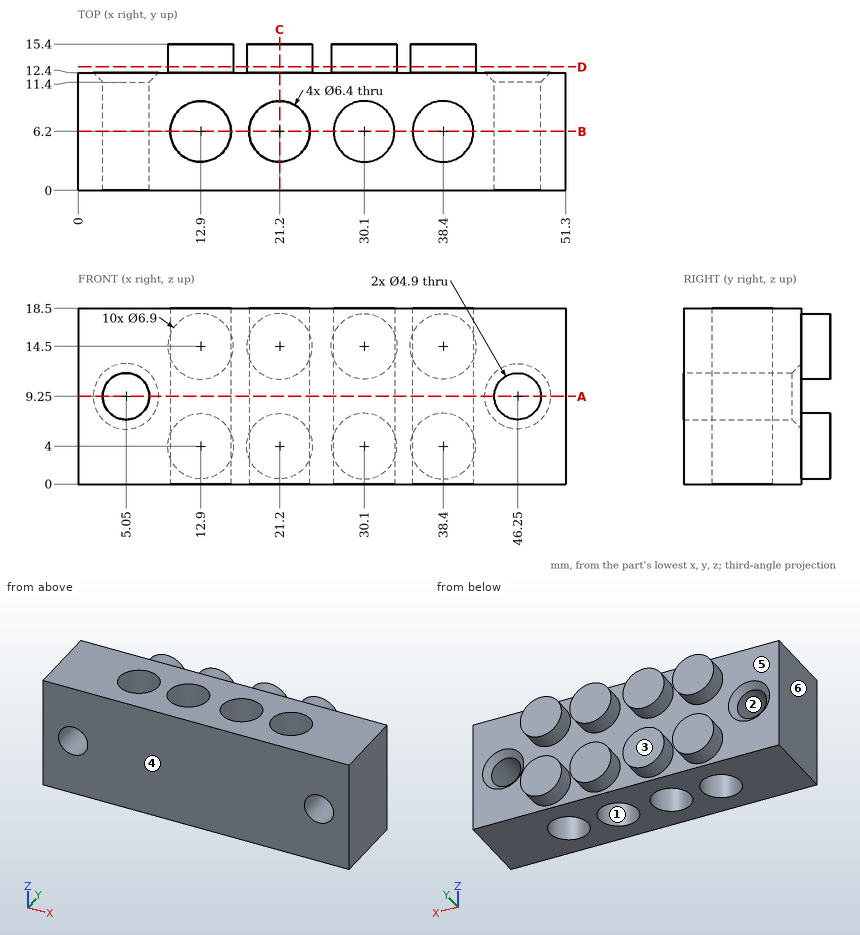
Study the drawing (mm; zero at the part's minimum x, y, z) and answer. A direction names the side the tool comes from. Coordinates: 2 decimals unless noted, no trailing zeros. Write each loop counter-clockwise with the first axis right and the second up, starting at its lowest first coordinate (ties: lowest second). Pieces come first, ordered by that corner, then holes. Notation, with made-up numbers: (21.25, -18.5) -> (71.25, -18.5) arc R12 cw to (71.25, -4.5) -> close; hole circle Ø8 at (35.25, 28). An arc over 180 degrees is marked (long way). Write item = value, one per line.
(1) Section D-D on y = 13 is taken. Write down the section's boundary in (x, z).
From the geometry:
outline = circle Ø6.9 at (12.9, 4); circle Ø6.9 at (12.9, 14.5); circle Ø6.9 at (21.2, 4); circle Ø6.9 at (21.2, 14.5); circle Ø6.9 at (30.1, 4); circle Ø6.9 at (30.1, 14.5); circle Ø6.9 at (38.4, 4); circle Ø6.9 at (38.4, 14.5)
(2) For a pull along Y with two mould halves and no side action, classify the marked faces 1, 2, 3 and 4 as +Y half, -Y half, draft (parallel to the pull), parting line (faces both ways), or undercut.
From the geometry:
face_1 = undercut
face_2 = draft
face_3 = +Y half
face_4 = -Y half
(3) Section C-C on x = 21.2 is taken. Write down the section's boundary in (y, z), plus the area to 3 significant figures.
From the geometry:
outline = (0, 0) -> (3, 0) -> (3, 18.5) -> (0, 18.5) -> close; (9.4, 0) -> (12.4, 0) -> (12.4, 0.55) -> (15.4, 0.55) -> (15.4, 7.45) -> (12.4, 7.45) -> (12.4, 11.05) -> (15.4, 11.05) -> (15.4, 17.95) -> (12.4, 17.95) -> (12.4, 18.5) -> (9.4, 18.5) -> close
area = 152 mm2
(4) Straight lines are drawn through the part: L1, parallel to X at y = 13.5, z = 4.25; L2, parallel to Y at x = 38.4, z = 14.75; L3, parallel to Z at x = 5.05, y = 7.25. For each, find the intervals that lie inside material, in ascending order. Write a range as from..to.
From the geometry:
L1 = 9.46..16.34, 17.76..24.64, 26.66..33.54, 34.96..41.84
L2 = 0..3, 9.4..15.4
L3 = 0..6.8, 11.7..18.5
(5) Which of the six approach directions +Z, -Z, +X, -X, +Y, -Y give full straight-line access (tool end or side, diameter ignored) to the marked faces 5 and 6?
From the geometry:
face_5 = +Y
face_6 = +Z, -Z, -X, +Y, -Y
(6) Section B-B on y = 6.2 is taken. Write down the section's boundary in (x, z).
From the geometry:
outline = (0, 0) -> (9.7, 0) -> (9.7, 18.5) -> (0, 18.5) -> close; (16.1, 0) -> (18, 0) -> (18, 18.5) -> (16.1, 18.5) -> close; (24.4, 0) -> (26.9, 0) -> (26.9, 18.5) -> (24.4, 18.5) -> close; (33.3, 0) -> (35.2, 0) -> (35.2, 18.5) -> (33.3, 18.5) -> close; (41.6, 0) -> (51.3, 0) -> (51.3, 18.5) -> (41.6, 18.5) -> close; hole circle Ø4.9 at (5.05, 9.25); hole circle Ø4.9 at (46.25, 9.25)
(7) Section A-A on z = 9.25 is taken. Write down the section's boundary in (x, y), plus the area to 3 significant figures.
From the geometry:
outline = (0, 0) -> (2.6, 0) -> (2.6, 11.4) -> (1.6, 12.4) -> (0, 12.4) -> close; (7.5, 0) -> (43.8, 0) -> (43.8, 11.4) -> (42.8, 12.4) -> (8.5, 12.4) -> (7.5, 11.4) -> close; (48.7, 0) -> (51.3, 0) -> (51.3, 12.4) -> (49.7, 12.4) -> (48.7, 11.4) -> close; hole circle Ø6.4 at (12.9, 6.2); hole circle Ø6.4 at (21.2, 6.2); hole circle Ø6.4 at (30.1, 6.2); hole circle Ø6.4 at (38.4, 6.2)
area = 384 mm2
